from build123d import *

# Parameters (mm, degrees)
SKETCH1_R                                            = 25.4
BOSS_EXTRUDE1_DEPTH                                  = 15.875
BOSS_EXTRUDE2_DEPTH                                  = 11.176
SKETCH3_W                                            = 12.7
SKETCH3_H                                            = 76.2
BOSS_EXTRUDE3_DEPTH                                  = 57.15
CBORE_FOR_3_8_BINDING_HEAD_MACHINE_SCREW_D           = 12.7
CBORE_FOR_3_8_BINDING_HEAD_MACHINE_SCREW_CBORE_D     = 35.052
CBORE_FOR_3_8_BINDING_HEAD_MACHINE_SCREW_CBORE_DEPTH = 1.524
BOSS_EXTRUDE7_DEPTH                                  = 5.588
F_25_64_0_45_DIAMETER_HOLE1_D                        = 11.43
FILLET1_R                                            = 6.35


with BuildPart() as part:
    # Sketch1 → Boss-Extrude1 (new body)
    with BuildSketch(Plane(origin=(0, 0, 0), x_dir=(1, 0, 0), z_dir=(0, 1, 0))):
        with Locations(Location((0, 0, 0), (0, 0, 270))):
            Circle(SKETCH1_R)
    extrude(amount=BOSS_EXTRUDE1_DEPTH)

    # Sketch2 → Boss-Extrude2 (add)
    with BuildSketch(Plane(origin=(0, 0, 0), x_dir=(1, 0, 0), z_dir=(0, 1, 0))):
        with BuildLine():
            Line((-88.9, 38.1), (-88.9, -38.1))
            Line((-88.9, -38.1), (0, -25.4))
            ThreePointArc((0, -25.4), (-25.4, 0), (0, 25.4))
            Line((0, 25.4), (-88.9, 38.1))
        make_face()
    extrude(amount=BOSS_EXTRUDE2_DEPTH)

    # Sketch3 → Boss-Extrude3 (add)
    with BuildSketch(Plane(origin=(0, 0, 0), x_dir=(1, 0, 0), z_dir=(0, 1, 0))):
        with Locations((-95.25, 0)):
            Rectangle(SKETCH3_W, SKETCH3_H)
    extrude(amount=BOSS_EXTRUDE3_DEPTH)

    # CBORE for 3/8 Binding Head Machine Screw1 (through all)
    with Locations(Plane.ZX.offset(15.875)):
        with Locations((0, 0)):
            CounterBoreHole(CBORE_FOR_3_8_BINDING_HEAD_MACHINE_SCREW_D / 2, CBORE_FOR_3_8_BINDING_HEAD_MACHINE_SCREW_CBORE_D / 2, CBORE_FOR_3_8_BINDING_HEAD_MACHINE_SCREW_CBORE_DEPTH)

    # Sketch10 → Boss-Extrude7 (add, symmetric)
    with BuildSketch(Plane.XY):
        Polygon((-88.9, 57.15), (-25.4, 15.875), (-22.86, 14.224), (-22.86, 11.176), (-88.9, 11.176), align=None)
    extrude(amount=BOSS_EXTRUDE7_DEPTH, both=True)

    # 25/64 (0.45) Diameter Hole1 (through all)
    with Locations(Plane(origin=(-88.9, 42.164, 23.7998), x_dir=(0, 0, 1), z_dir=(1, 0, 0))):
        with Locations((0, 0), (-47.625, 0)):
            Hole(F_25_64_0_45_DIAMETER_HOLE1_D / 2)

    # Fillet1
    fillet1_edges = [part.edges().sort_by_distance(p)[0] for p in [
        (-95.25, 57.15, -38.1),
        (-95.25, 57.15, 38.1),
    ]]
    fillet(fillet1_edges, radius=FILLET1_R)


solid = part.part
The listing builds one solid part. Answer for the finished solid, in the listing's coordinates (mm). A direction names the side the tool comes from. Round coordinates to 2 decimals unless told otherwise and drop trailing zeros. Write each loop counter-clockwise with the first axis right and the second up, starting at its lowest first coordinate (ties: lowest second). Pieces come first, ordered by that corner, then holes. Notation, with made-up numbers: (80, 33) - (121, 33) arc R31 cw to (121, 60) - close; hole circle Ø4 at (-7, -12). An arc over 180 degrees is marked (long way). Use a Markdown table: item, result. Add a question column.
1. Consider line 1 (X direction, y = 10, z = 0); line 2 (X direction, y = 15.2, z = 0); line 3 (Y direction, x = -67, z = -22). Determine where each line is inside the solid, lowest interval first.
2. The part is cut by section D-D (x = -9). Write down the section's boundary in (y, z) (3 decimals), and give its area (3 significant figures).
3. The part is cut by section C-C (z = -15). Write down the section's boundary in (x, y) (3 decimals), and give its area (3 significant figures).
4. The part is cut by section A-A (y = 32). Write down the section's boundary in (x, z).
5. A tool of negligible diameter and unlimited length cuts with its end or side. For faces 1 (the face through (-55, 11.176, -18)), 2 (the face through (-64, 29, 5.588)), 3 (the face through (-95.16, 55.34, 36.19)), 4 (the face through (-95, 25, 38.1)), 5 (the face through (5.26, 15.12, 16.72)), from which of +Z, -Z, +X, -X, +Y, -Y can it reach the whole face along a straight path? Write none if from no direction.
6. For a pull along Y with two mould halves and no side action, classify faces 6 (the face through (-45.07, 5.51, 31.84)), 7 (the face through (-56.39, 36.02, 0.08)), 8 (the face through (-95.339, 47.743, 25.039)) as +Y half, -Y half, draft (parallel to the pull), parting line (faces both ways), or undercut.
7. Flat-ended cylindrical pins translate along their axes: P1, Ø8, axis at x = -70.5, y = 9, coming from the -Z side; P2, Ø1, axis at x = -23, y = 9, coming from the -Z side; P3, Ø14.5, axis at x = 0, z = 0, coming from the -Y side; P4, Ø1.5, axis at x = -15.5, z = 9, coming from the +Y side (3 decimals). Find the tip coordinate at first contact, or state that the pin passes through.
8. The part is cut by section B-B (x = -45). Write down the section's boundary in (y, z) (3 decimals), and give its area (3 significant figures).
Reported:
| question | item | result |
|---|---|---|
| 1 | line 1 | -101.6 to -6.35, 6.35 to 25.4 |
| 1 | line 2 | -101.6 to -17.53, 17.53 to 25.4 |
| 1 | line 3 | 0 to 11.18 |
| 2 | outline | (0, -26.686) - (11.176, -26.686) - (11.176, -23.752) - (15.875, -23.752) - (15.875, -15.039) - (14.351, -15.039) - (14.351, 15.039) - (15.875, 15.039) - (15.875, 23.752) - (11.176, 23.752) - (11.176, 26.686) - (0, 26.686) - close |
| 2 | area | 774 mm^2 |
| 3 | outline | (-101.6, 0) - (20.498, 0) - (20.498, 15.875) - (9.064, 15.875) - (9.064, 14.351) - (-9.064, 14.351) - (-9.064, 15.875) - (-20.498, 15.875) - (-20.498, 11.176) - (-88.9, 11.176) - (-88.9, 57.15) - (-101.6, 57.15) - close |
| 3 | area | 2,110 mm^2 |
| 4 | outline | (-101.6, -38.1) - (-88.9, -38.1) - (-88.9, -5.59) - (-50.21, -5.59) - (-50.21, 5.59) - (-88.9, 5.59) - (-88.9, 38.1) - (-101.6, 38.1) - close |
| 5 | face 1 | -Z, +Y |
| 5 | face 2 | +Z, +Y |
| 5 | face 3 | +Z, +X, -X, +Y |
| 5 | face 4 | +Z, +X, -X, +Y, -Y |
| 5 | face 5 | +Y |
| 6 | face 6 | draft |
| 6 | face 7 | +Y half |
| 6 | face 8 | undercut |
| 7 | P1 | z = -36.04 |
| 7 | P2 | z = -28.76 |
| 7 | P3 | y = 0 |
| 7 | P4 | y = 15.875 |
| 8 | outline | (0, -31.829) - (11.176, -31.829) - (11.176, -5.588) - (28.615, -5.588) - (28.615, 5.588) - (11.176, 5.588) - (11.176, 31.829) - (0, 31.829) - close |
| 8 | area | 906 mm^2 |
